Source: three-view drawing plus pictorial views. Frame: mm from the lowest corner of the part. A direction names the side the tool comes from. Give positions to 0.01 mm unless a question says otherwise; leave off trailing zeros. Order: outer loops, then holes, each group sorted by start corner. A loop starts at its lowest first (then second) coordinate and runs counter-clockwise, first axis right, second up.
1) Section C-C, the plane z = 14. Return loops of the section in (x, y), plus the area to 3 significant figures.
2) Access query for the marked faces 1 and 2. Directions: +Z, -Z, +X, -X, +Y, -Y. A direction counts if a zero-diameter tool reaches every point of the face in a straight line with its end or side. Return the directions, or none.
3) Section D-D, the plane y = 65. Return loops of the section in (x, z).
4) Material intervals for line 1 (Z direction, x = 69.5, y = 15.75); line 2 (X direction, y = 8.5, z = 5.5); line 3 (Y direction, x = 9, z = 25.5), sorted ascending.
5) Section A-A, the plane z = 5.5. Return loops of the section in (x, y), plus the area to 3 significant figures.
6) Section B-B, the plane x = 69.5. Return loops of the section in (y, z), plus the area to 3 significant figures.
7) First-contact query: P1, Ø17, axis at y = 74, z = 21.5, coming from the -X side; P2, Ø6, axis at x = 32, z = 32.5, coming from the +Y side; P3, Ø1.5, axis at x = 70, z = 41, coming from the -Y side. Flat tips, straight axial feed; report the tip coordinate or a pass-through.
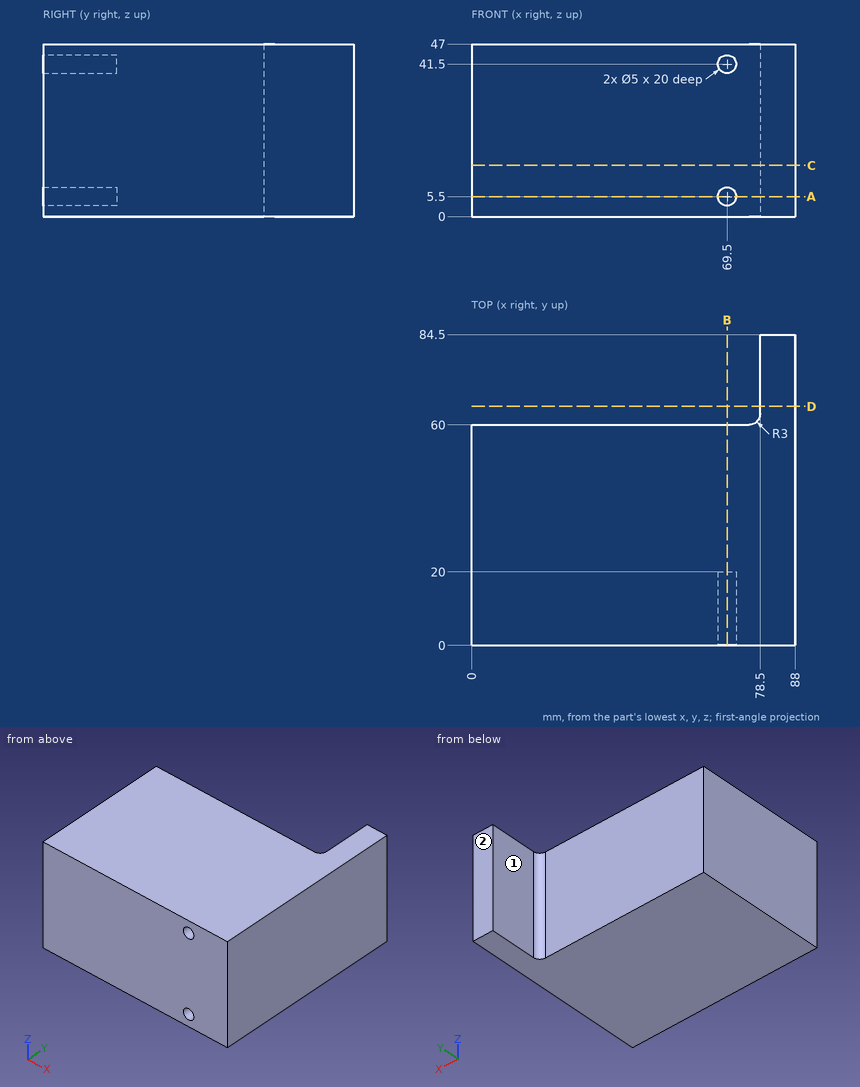
From the geometry:
1. outline: (0, 0) - (88, 0) - (88, 84.5) - (78.5, 84.5) - (78.5, 63) arc R3 cw to (75.5, 60) - (0, 60) - close
1. area: 5,510 mm2
2. face 1: +Z, -Z, -X, +Y
2. face 2: +Z, -Z, +X, -X, +Y
3. outline: (78.5, 0) - (88, 0) - (88, 47) - (78.5, 47) - close
4. line 1: z = 0 to 3, 8 to 39, 44 to 47
4. line 2: x = 0 to 67, 72 to 88
4. line 3: y = 0 to 60
5. outline: (0, 0) - (67, 0) - (67, 20) - (72, 20) - (72, 0) - (88, 0) - (88, 84.5) - (78.5, 84.5) - (78.5, 63) arc R3 cw to (75.5, 60) - (0, 60) - close
5. area: 5,410 mm2
6. outline: (0, 0) - (60, 0) - (60, 47) - (0, 47) - (0, 44) - (20, 44) - (20, 39) - (0, 39) - (0, 8) - (20, 8) - (20, 3) - (0, 3) - close
6. area: 2,620 mm2
7. P1: stops at x = 78.5
7. P2: stops at y = 60
7. P3: stops at y = 20
